from build123d import *

# Parameters (mm, degrees)
SKETCH1_R           = 20
SKETCH1_R_2         = 10
BOSS_EXTRUDE2_DEPTH = 50
BOSS_EXTRUDE3_REACH = 87
SKETCH4_W           = 32
SKETCH4_H           = 20
SKETCH5_R           = 11.161512364
CUT_EXTRUDE1_DEPTH  = 25
SKETCH7_W           = 4.481872956
SKETCH7_H           = 18.163379873
CUT_EXTRUDE2_DEPTH  = 51
SKETCH9_R           = 5
CUT_EXTRUDE3_DEPTH  = 21
CUT_EXTRUDE4_START  = 19
SKETCH10_W          = 12.248004276
SKETCH10_H          = 7.5
CUT_EXTRUDE4_DEPTH  = 15
SKETCH11_R          = 3
CUT_EXTRUDE5_DEPTH  = 25


with BuildPart() as part:
    # Sketch1 → Boss-Extrude2 (new body)
    with BuildSketch(Plane.XY):
        Circle(SKETCH1_R)
        Circle(SKETCH1_R_2, mode=Mode.SUBTRACT)
    extrude(amount=BOSS_EXTRUDE2_DEPTH)

    # Sketch4 → Boss-Extrude3 (add, up to next)
    with BuildSketch(Plane(origin=(0, 65, 0), x_dir=(1, 0, 0), z_dir=(0, 1, 0)), mode=Mode.PRIVATE) as boss_extrude3_sk1:
        with Locations((0, -40)):
            Rectangle(SKETCH4_W, SKETCH4_H)
    boss_extrude3_tool1 = extrude(boss_extrude3_sk1.sketch, amount=-BOSS_EXTRUDE3_REACH, mode=Mode.PRIVATE) - part.part
    add(boss_extrude3_tool1.solids().sort_by_distance((0, 65, 40))[0])

    # Sketch5 → Cut-Extrude1 (cut)
    with BuildSketch(Plane(origin=(0, 65, 0), x_dir=(1, 0, 0), z_dir=(0, 1, 0))):
        with Locations((0, -28.900111213)):
            Circle(SKETCH5_R)
    extrude(amount=-CUT_EXTRUDE1_DEPTH, mode=Mode.SUBTRACT)

    # Sketch7 → Cut-Extrude2 (cut, through all)
    with BuildSketch(Plane(origin=(0, 0, 0), x_dir=(-1, 0, 0), z_dir=(0, 0, -1))):
        with Locations((0, -15.183116037)):
            Rectangle(SKETCH7_W, SKETCH7_H)
    extrude(amount=-CUT_EXTRUDE2_DEPTH, mode=Mode.SUBTRACT)

    # Sketch9 → Cut-Extrude3 (cut, through all)
    with BuildSketch(Plane(origin=(0, 0, 30), x_dir=(-1, 0, 0), z_dir=(0, 0, -1))):
        with Locations((0, 28.274780399)):
            Circle(SKETCH9_R)
    extrude(amount=-CUT_EXTRUDE3_DEPTH, mode=Mode.SUBTRACT)

    # Sketch10 → Cut-Extrude4 (cut)
    with BuildSketch(Plane(origin=(0, 0, 0), x_dir=(0, 0, -1), z_dir=(1, 0, 0)).offset(CUT_EXTRUDE4_START)):
        with Locations((-25, -14.823528739)):
            Rectangle(SKETCH10_W, SKETCH10_H)
    cut_extrude4 = extrude(amount=-CUT_EXTRUDE4_DEPTH, mode=Mode.SUBTRACT)

    # Mirror1: Cut-Extrude4 across plane
    add(cut_extrude4.mirror(Plane(origin=(0, 0, 0), x_dir=(0, 0, 1), z_dir=(1, 0, 0))), mode=Mode.SUBTRACT)

    # Sketch11 → Cut-Extrude5 (cut, through all)
    with BuildSketch(Plane.ZY.offset(4)):
        with Locations((25, -14.823528739)):
            Circle(SKETCH11_R)
    extrude(amount=-CUT_EXTRUDE5_DEPTH, mode=Mode.SUBTRACT)


solid = part.part
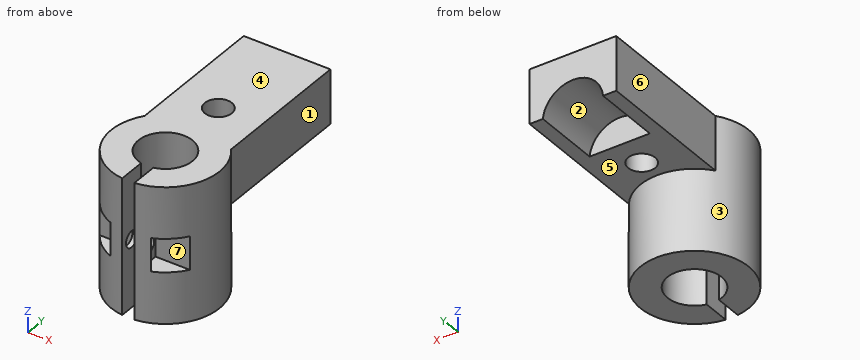
Verification items for the finished model (mm, model axes). Face numbers are marked on the shaded views. A direction names the side the tool comes from. Coordinates: 2 decimals unless noted, no trailing zeros. Write each loop counter-clockwise with the first axis right and the second up, starting at its lowest first coordinate (ties: lowest second). Pieces come first, ordered by that corner, then holes. Notation, with made-up numbers: (75, -8) - (125, -8) arc R14 cw to (125, 6) - close; hole circle Ø7 at (-19, 59). An arc over 180 degrees is marked (long way). Answer as a JSON object with one key per item and string values.
(1) Cross-section at C-C on z = 25. Record the cut outline in (x, y).
Report:
{"outline": "(-16.65, -11.07) - (-4, -11.07) - (-4, -11.82) - (-2.24, -11.82) - (-2.24, -9.75) arc R10 cw (long way) to (2.24, -9.75) - (2.24, -11.82) - (4, -11.82) - (4, -11.07) - (16.65, -11.07) arc R20 ccw (long way) to start; (-7.42, -18.57) arc R20 ccw to (-2.24, -19.87) - (-2.24, -17.82) - (-4, -17.82) - (-4, -18.57) - close; (2.24, -19.87) arc R20 ccw to (7.42, -18.57) - (4, -18.57) - (4, -17.82) - (2.24, -17.82) - close"}
(2) Cross-section at A-A on x = 0. Record the cut outline in (y, z), plus the area to 3 significant figures.
Report:
{"outline": "(10, 0) - (20, 0) - (20, 30) - (23.27, 30) - (23.27, 50) - (10, 50) - close; (33.27, 30) - (40, 30) - (40, 40.06) - (65, 40.06) - (65, 50) - (33.27, 50) - close", "area": "948 mm^2"}
(3) Gauge pin test, flat ends, axial feed: pin 1 Ø22 at (y, z) = (34.5, 43) entering from +X; pin 2 Ø3 at (x, y) = (-12.5, 54.5) entering from -Z; pin 3 Ø10 at (y, z) = (35.5, 42) entering from -X. Record the tip position at first contact, or that the pin passes through.
Report:
{"pin 1": "x = 16", "pin 2": "z = 30", "pin 3": "x = -16"}
(4) Thickness scan on line 1 along Y through (x, z) = (0, 37); line 2 along X through (y, z) = (28, 48.5); line 3 along X through (y, z) = (0, 35.5). Record the ranges inside material, lowest first.
Report:
{"line 1": "10 to 23.27, 33.27 to 40", "line 2": "-16 to -4.99, 4.99 to 16", "line 3": "-20 to -10, 10 to 20"}
(5) Cross-section at D-D on x = 6. Record the cut outline in (y, z), plus the area to 3 significant figures.
Report:
{"outline": "(-19.08, 0) - (-8, 0) - (-8, 50) - (-19.08, 50) - close; (8, 0) - (19.08, 0) - (19.08, 30) - (40, 30) - (40, 38.31) - (65, 38.31) - (65, 50) - (8, 50) - close; hole (-18.57, 18.88) - (-11.07, 18.88) - (-11.07, 31.12) - (-18.57, 31.12) - close", "area": "1,730 mm^2"}
(6) Mould release check, pull along Z, two halves, no side actions. Record for the marked faces 4, 5, 6 and 7: pulls with the +Z half, pulls with the -Z half, needs draft (parallel to the pull), parting line crosses it, or undercut.
Report:
{"face 4": "pulls with the +Z half", "face 5": "pulls with the -Z half", "face 6": "needs draft", "face 7": "undercut"}
(7) Tool access check on the marked faces 1, 2 and 3. Record the directions out of +Z, -Z, +X, -X, +Y, -Y that give a thin tool (end or side, any length) a straight path to the whole face; none if there is none.
Report:
{"face 1": "+Z, -Z, +X, +Y", "face 2": "-Z, +Y", "face 3": "-Z"}
(8) Cross-section at B-B on y = 0. Record the cut outline in (x, z).
Report:
{"outline": "(-20, 0) - (-10, 0) - (-10, 50) - (-20, 50) - close; (10, 0) - (20, 0) - (20, 50) - (10, 50) - close"}
